CAD build for the part. Positions are in the model's coordinates, mm. Face numbers are marked on the shaded views. A direction names the side the tool comes from. Round coordinates to 2 decimals unless told otherwise and drop trailing zeros. Write each loop counter-clockwise with the first axis right and the second up, starting at its lowest first coordinate (ties: lowest second). Pieces come first, ordered by that corner, then holes. Notation, with made-up numbers: (48, 78.25) -> (80, 78.25) arc R38 cw to (80, 117.25) -> close; hole circle Ø6 at (-12, 41.25). An arc over 180 degrees is marked (long way). Put each result on its own line as item: value. Start each with the question number.
1. Saw through at D-D on z = 4.5. List the corners of the cut face in (x, y).
2. Saw through at C-C on z = 1. List the corners of the cut face in (x, y), and give its area (3 significant figures).
3. 3-axis set-ups, long thin cutter, end or side, ignore diameter. For the marked faces 1 and 2: which of +Z, -Z, +X, -X, +Y, -Y reach the whole face in a straight line?
4. Flat gauge pins, fed straight in: P1, Ø4, axis at x = 0.5, y = 35, coming from the +Z side; P2, Ø1, axis at x = -2, z = -4.5, coming from the +Y side; P3, Ø6, axis at y = 50.5, z = -1, coming from the -X side. Where does each tip first touch, or does it go through?
5. Saw through at A-A on x = 0. List the corners of the cut face in (y, z), and give its area (3 significant figures).
6. Saw through at B-B on y = 63. List the corners of the cut face in (x, z), and give its area (3 significant figures).
7. Drill centre lines: line 1 (Y direction, x = 2.5, z = 3.25); line 2 (X direction, y = 80, z = -0.25); line 3 (Z direction, x = -1, y = 15). Where is each one in solid material? Low to high. Write a range as from..to.
Autodesk Inventor part; units mm, degrees
ref_plane "YZ Plane" through (0, 0, 0) normal (1, 0, 0) x (0, 1, 0)
ref_plane "XZ Plane" through (0, 0, 0) normal (0, 1, 0) x (-1, 0, 0)
ref_plane "XY Plane" through (0, 0, 0) normal (0, 0, 1) x (1, 0, 0)
sketch "Sketch1" plane through (0, 0, 0) normal (0, 1, 0) x (-1, 0, 0)
  circle A0 centre (0, 0) radius 7.5
  dimension "d0" = 15
extrude "Extrusion1" add sketch "Sketch1" along normal blind 5
sketch "Sketch2" plane through (0, 5, 0) normal (0, 1, 0) x (1, 0, 0)
  circle A0 centre (0, 0) radius 2.5
  dimension "d3" = 5
extrude "Extrusion2" add sketch "Sketch2" along normal blind 80
thread "Thread1"
sketch "Sketch3" plane through (0, 0, 0) normal (0, -1, 0) x (1, 0, 0)
  circle A0 centre (0, 0) radius 7.5
  line L0 (-7.5, 0) -> (0, 0)
  line L1 (0, 0) -> (-3.75, -6.4952)
  line L2 (0, 0) -> (3.75, -6.4952)
  line L3 (0, 0) -> (7.5, 0) construction
  line L4 (0, 0) -> (3.75, 6.4952)
  line L5 (0, 0) -> (7.5, 0) construction
  line L6 (0, 0) -> (-3.75, 6.4952)
  line L7 (0, 0) -> (7.5, 0) construction
  line L8 (-7.5, 0) -> (-3.75, -6.4952)
  line L9 (-3.75, -6.4952) -> (3.75, -6.4952)
  line L10 (3.75, -6.4952) -> (7.5, 0)
  line L11 (7.5, 0) -> (3.75, 6.4952)
  line L12 (3.75, 6.4952) -> (-3.75, 6.4952)
  line L13 (-3.75, 6.4952) -> (-7.5, 0)
  point P0 (7.5, 0)
  point P1 (7.5, 0)
  dimension "d8" = 60
  dimension "d9" = 60
  dimension "d10" = 60
  dimension "d11" = 120
extrude "Extrusion3" cut sketch "Sketch3" against normal through all contours L11 A0 | A0 L10 | L12 A0 | A0 L9 | L13 A0 | A0 L8
properties part number "Bolt" material "Steel, Mild"
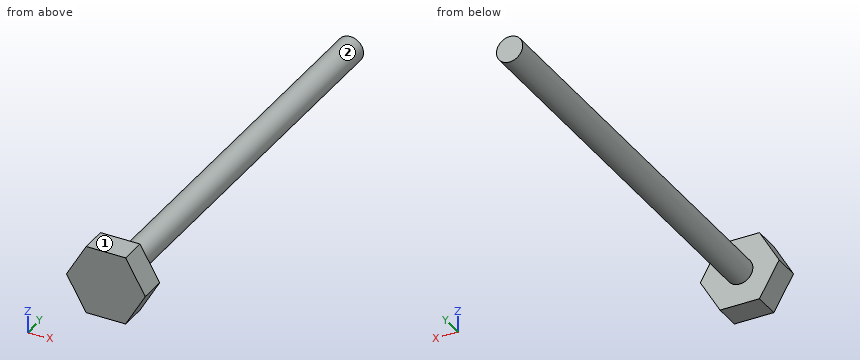
Return value:
1. outline: (-4.9, 0) -> (4.9, 0) -> (4.9, 5) -> (-4.9, 5) -> close
2. outline: (-6.92, 0) -> (6.92, 0) -> (6.92, 5) -> (2.29, 5) -> (2.29, 85) -> (-2.29, 85) -> (-2.29, 5) -> (-6.92, 5) -> close
2. area: 436 mm^2
3. face 1: +Z, +X, -X, +Y, -Y
3. face 2: +Y
4. P1: stops at z = 2.5
4. P2: stops at y = 5
4. P3: stops at x = -2.5
5. outline: (0, -6.5) -> (5, -6.5) -> (5, -2.5) -> (85, -2.5) -> (85, 2.5) -> (5, 2.5) -> (5, 6.5) -> (0, 6.5) -> close
5. area: 465 mm^2
6. outline: circle Ø5 at (0, 0)
6. area: 19.6 mm^2
7. line 1: y = 0..5
7. line 2: x = -2.49..2.49
7. line 3: z = -2.29..2.29
